from build123d import *

# Parameters (mm, degrees)
BOSS_EXTRUDE1_DEPTH        = 80
F_3_5_3_5_DIAMETER_HOLE1_D = 3.5


with BuildPart() as part:
    # Sketch1 → Boss-Extrude1 (new body)
    with BuildSketch(Plane.XY):
        Polygon((6, -2.8), (6, 0), (0, 0), (0, -19), (2, -19), (2, -14.384515279), (1.334, -14), (2, -13.615484721), (2, -9), (6, -9), (6, -6.2), (4.5, -6.2), (4.5, -7.35), (1.5, -7.35), (1.5, -1.65), (4.5, -1.65), (4.5, -2.8), align=None)
    extrude(amount=-BOSS_EXTRUDE1_DEPTH)

    # Ø3.5 (3.5) Diameter Hole1 (through all)
    with Locations(Plane.ZY):
        with Locations((-10, -14), (-70, -14)):
            Hole(F_3_5_3_5_DIAMETER_HOLE1_D / 2)


solid = part.part
Can you work these out from the model? Positions are in its coordinate system, mm. A direction names the side the tool comes from. Give positions to 0.01 mm unless a question says otherwise; leave off trailing zeros. Loops run counter-clockwise (first coordinate to the right, second up) from the corner with the lowest first, then second, coordinate; pieces in that order, holes last. Notation, with made-up numbers: M 58.25,-28.75 L 117.25,-28.75 A12 cw 117.25,-19.75 Z; hole C -18,7.5 d7. An arc over 180 degrees is marked long. One line per item, written item: value. Start each with the question number.
1) If I drill on line 1 (Z direction, x = 0.55, y = -14); line 2 (Y direction, x = 1.35, z = -70); line 3 (Y direction, x = 5.1, z = -14.5), over which ranges is the centre line in solid material (lowest first)? Write a range as [from, to].
2) If we section it at C-C, the plane z = -46: Write out the boundary of the cut face in (x, y), and give its area (3 significant figures).
3) On a 3-axis mill with a long thin cutter (end or side, diameter ignored), from which of +Z, -Z, +X, -X, +Y, -Y can I reach the whole of each face in a straight line? I mean faces 5 (the face through (6, -8, -39)), 6 (the face through (2, -11, -39)), 7 (the face through (3, -7.35, -39)), 8 (the face through (5, -2.8, -39)), 9 (the face through (1, -7, 0)). Say none if no direction works.
4) Thinking about a two-plate mould opening in X: for faces 1 (the face through (0, -9, -39)), 2 (the face through (1.5, -5, -39)), 3 (the face through (3, 0, -39)), 4 (the face through (3, -1.65, -39)), which applies, +X half, -X half, draft (parallel to the pull), parting line (faces both ways), or undercut?
5) If we section it at A-A, the plane z = -70: Write out the boundary of the cut face in (x, y), and give its area (3 significant figures).
6) If we section it at B-B, the plane x = 2.9: Write out the boundary of the cut face in (y, z), and give its area (3 significant figures).
7) If we section it at D-D, the plane y = -3.5: Write out the boundary of the cut face in (x, z).
8) I'm going to push flat-ended pins straight in: pin 1 (2.5 mm diameter, centred on y = -16, z = -49.5, fed in from +X); pin 2 (0.8 mm diameter, centred on x = 5.5, z = -50, fed in from -Y). Where does each tip first touch, or does it pass through?
Completed:
1. line 1: z = [-80, -71.75], [-68.25, -11.75], [-8.25, 0]
1. line 2: y = [-19, -15.75], [-12.25, 0]
1. line 3: y = [-9, -6.2], [-2.8, 0]
2. outline: M 0,-19 L 2,-19 L 2,-14.38 L 1.33,-14 L 2,-13.62 L 2,-9 L 6,-9 L 6,-6.2 L 4.5,-6.2 L 4.5,-7.35 L 1.5,-7.35 L 1.5,-1.65 L 4.5,-1.65 L 4.5,-2.8 L 6,-2.8 L 6,0 L 0,0 Z
2. area: 51.5 mm^2
3. face 5: +Z, -Z, +X, +Y, -Y
3. face 6: +Z, -Z, +X, -Y
3. face 7: +Z, -Z
3. face 8: +Z, -Z, +X
3. face 9: +Z, +X, -X, +Y, -Y
4. face 1: -X half
4. face 2: undercut
4. face 3: draft
4. face 4: undercut
5. outline: M 0,-19 L 2,-19 L 2,-15.75 L 0,-15.75 Z; M 0,-12.25 L 2,-12.25 L 2,-9 L 6,-9 L 6,-6.2 L 4.5,-6.2 L 4.5,-7.35 L 1.5,-7.35 L 1.5,-1.65 L 4.5,-1.65 L 4.5,-2.8 L 6,-2.8 L 6,0 L 0,0 Z
5. area: 44.8 mm^2
6. outline: M -9,-80 L -7.35,-80 L -7.35,0 L -9,0 Z; M -1.65,-80 L 0,-80 L 0,0 L -1.65,0 Z
6. area: 264 mm^2
7. outline: M 0,-80 L 1.5,-80 L 1.5,0 L 0,0 Z
8. pin 1: stops at x = 2
8. pin 2: stops at y = -9
